Input: dimensioned drawing with shaded views. Units: mm. Origin: part minimum x, y, z. Coordinates: 2 decimals unless noted, no trailing zeros. Order: outer loops, then holes, each group sorted by start corner. A loop starts at its lowest first (then second) coordinate and runs counter-clockwise, first axis right, second up. Notation, with made-up numbers: (24.25, -37) -> (39.25, -37) arc R8 ccw to (39.25, -31) -> close; hole circle Ø10 at (-27.75, -25). An arc over 180 degrees is marked (long way). Put each result on its own line as item: value.
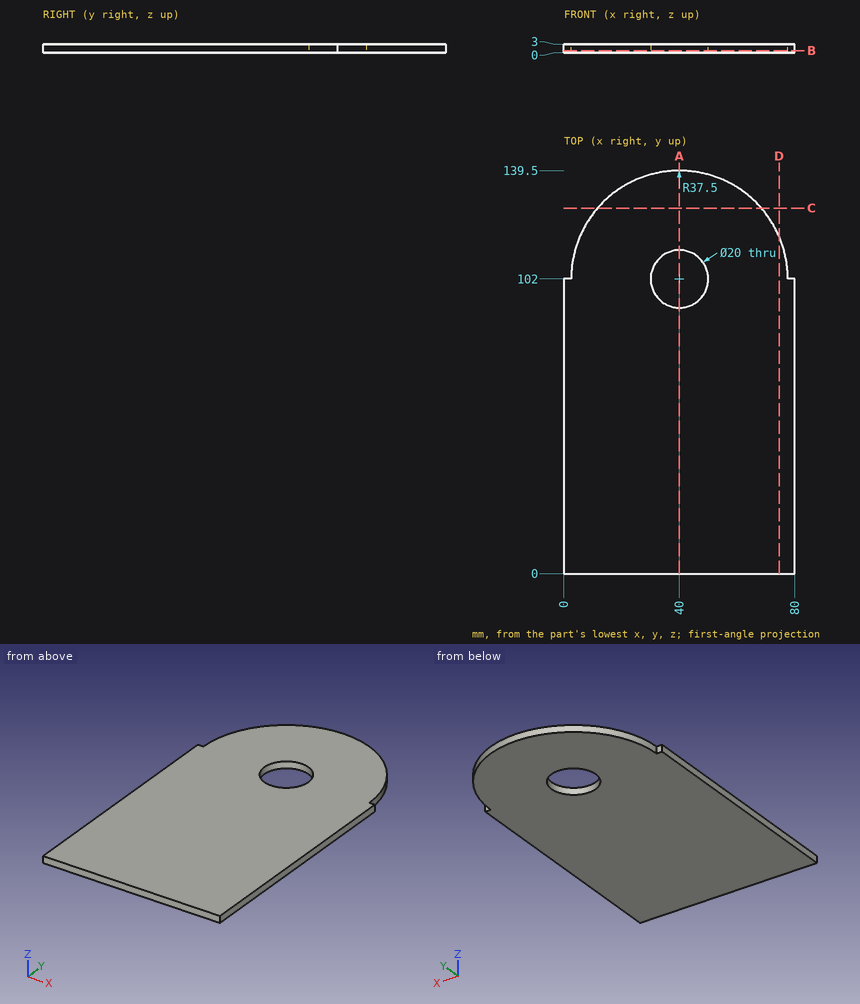
1. Cut plane A-A on x = 40. Output: boundary loops of the cut face in (y, z), plus the area to 4 significant figures.
Numbers:
outline: (0, 0) -> (92, 0) -> (92, 3) -> (0, 3) -> close; (112, 0) -> (139.5, 0) -> (139.5, 3) -> (112, 3) -> close
area: 358.5 mm2
2. Cut plane B-B on z = 0.7. Output: boundary loops of the cut face in (x, y), plus the area to 3 significant figures.
Numbers:
outline: (0, 0) -> (80, 0) -> (80, 102) -> (77.5, 102) arc R37.5 ccw to (2.5, 102) -> (0, 102) -> close; hole circle Ø20 at (40, 102)
area: 10,100 mm2
3. First-contact query: pin 1 (1.2 mm diameter, centred on x = 1, z = 1, fed in from +Y); pin 2 (12 mm diameter, centred on x = 40, y = 102, fed in from -Z). Flat tips, straight axial feed; report the tip coordinate or a pass-through.
Numbers:
pin 1: stops at y = 102
pin 2: passes through
4. Cut plane C-C on y = 126.5. Output: boundary loops of the cut face in (x, z).
Numbers:
outline: (11.61, 0) -> (68.39, 0) -> (68.39, 3) -> (11.61, 3) -> close
5. Ray query, line 1 along Y through (x, z) = (40, 1.5); line 2 along Y through (x, z) = (11, 2.6); line 3 along Y through (x, z) = (32, 1.45). Return the intervals inside material, ascending.
Numbers:
line 1: y = 0 to 92, 112 to 139.5
line 2: y = 0 to 125.77
line 3: y = 0 to 96, 108 to 138.64
6. Cut plane D-D on x = 74.5. Output: boundary loops of the cut face in (y, z).
Numbers:
outline: (0, 0) -> (116.7, 0) -> (116.7, 3) -> (0, 3) -> close
